The model under review builds one solid part; all positions refer to its coordinate system, in mm. A direction names the side the tool comes from. Give positions to 0.01 mm unless a question says otherwise; leave off trailing zeros. Write each loop counter-clockwise with the first axis right and the second up, starting at its lowest first coordinate (ties: lowest second). Pieces come first, ordered by that corner, then holes. Notation, with made-up numbers: M -14,15 L 18,15 A19 ccw 18,46 Z; hole C -2,-1.5 d5. An arc over 180 degrees is marked long. Write item = value, one per line. Start each with the question number.
```python
from build123d import *


with BuildPart() as part:
    # Sketch1 → Revolve1 (revolve)
    with BuildSketch(Plane.XY):
        Polygon((12.3444, 4.699), (11.0744, 4.699), (11.0744, 3.81), (0, 3.81), (0, 3.302), (10.16, 3.302), (10.16, 2.5), (12.3444, 2.5), align=None)
    revolve(axis=Axis((0, 0, 0), (1, 0, 0)))

    # Sketch7 → Revolve4 (revolve)
    with BuildSketch(Plane.XY):
        with BuildLine():
            Line((10.16, 3.302), (9.2837, 3.302))
            Line((9.2837, 3.302), (9.2837, 0))
            Line((9.2837, 0), (12.86069262, 0))
            Line((12.86069262, 0), (15.36069262, 0))
            ThreePointArc((15.36069262, 0), (14.628459573, 1.767766953), (12.86069262, 2.5))
            Line((12.86069262, 2.5), (10.16, 2.5))
            Line((10.16, 2.5), (10.16, 3.302))
        make_face()
    revolve(axis=Axis((12.86069262, 0, 0), (1, 0, 0)))


solid = part.part
```
Item 1: To check wall thickness, follow probe 1 along Z at (x, y) = (5.5, 0); probe 2 along Y at (x, z) = (0.5, -0.5); probe 3 along X at (y, z) = (-2, -1.75). State the ranges of each line that lie inside material, in increasing order. Write a range as [from, to].
Item 2: We need section B-B, the plane y = 2. Write out the cut boundary in (x, z), and give its area (3 significant figures).
Item 3: For faces 1 (the cylindrical face through (5.46, -0.83, -3.72)), 2 (the cylindrical face through (12.6, -0.54, -2.44)), 3 (the flat face through (0, -3, 2)), list the 3-axis set-ups (+Z, -Z, +X, -X, +Y, -Y) from which the entire face can be reached by the end or side of a thin tool; tool diameter is ignored.
Item 4: We need section A-A, the plane z = 0. Write out the cut boundary in (x, y).
Item 5: We need section C-C, the plane x = 11.25. Write out the cut boundary in (y, z), and give its area (3 significant figures).
Item 6: We need section D-D, the plane x = 2.5. Write out the cut boundary in (y, z), and give its area (3 significant figures).
Item 7: The part is to be moulded in two halves that separate along Y. For faces 4 (the cylindrical face through (11.7, -0.61, 4.66)), 5 (the flat face through (11.074, 0, 4)), 6 (the cylindrical face through (4.71, 3.05, -1.26)), say which applies: released by +Y, released by -Y, zero draft, split by the parting line, or undercut.
Item 8: Clearance check with flat-ended pins moving along their axes: P1, Ø4, axis at y = 1.5, z = -3.5, coming from the +X side; P2, Ø1.5, axis at x = 8.5, y = 2.5, coming from the +Z side; P3, Ø3.5, axis at y = 0, z = 0, coming from the -X side; P4, Ø5, axis at y = -3, z = 2, coming from the -X side. State where each tip first meets the part, or that it passes through.
Worked out:
q1.probe_1 = [-3.81, -3.3], [3.3, 3.81]
q1.probe_2 = [-3.78, -3.26], [3.26, 3.78]
q1.probe_3 = [9.28, 12.34]
q2.outline = M 0,-3.24 L 11.07,-3.24 L 11.07,-4.25 L 12.34,-4.25 L 12.34,-1.5 L 12.86,-1.5 A1.5 ccw 12.86,1.5 L 12.34,1.5 L 12.34,4.25 L 11.07,4.25 L 11.07,3.24 L 0,3.24 L 0,2.63 L 9.28,2.63 L 9.28,-2.63 L 0,-2.63 Z
q2.area = 38.9 mm²
q3.face_1 = -X
q3.face_2 = +X
q3.face_3 = +Z, -Z, -X, +Y, -Y
q4.outline = M 0,-3.81 L 11.07,-3.81 L 11.07,-4.7 L 12.34,-4.7 L 12.34,-2.5 L 12.86,-2.5 A2.5 ccw 12.86,2.5 L 12.34,2.5 L 12.34,4.7 L 11.07,4.7 L 11.07,3.81 L 0,3.81 L 0,3.3 L 9.28,3.3 L 9.28,-3.3 L 0,-3.3 Z
q5.outline = C 0,0 d9.4
q5.area = 69.4 mm²
q6.outline = C 0,0 d7.62; hole C 0,0 d6.6
q6.area = 11.4 mm²
q7.face_4 = split by the parting line
q7.face_5 = zero draft
q7.face_6 = undercut
q8.P1 = 14.59
q8.P2 = 3.38
q8.P3 = 9.28
q8.P4 = 0
